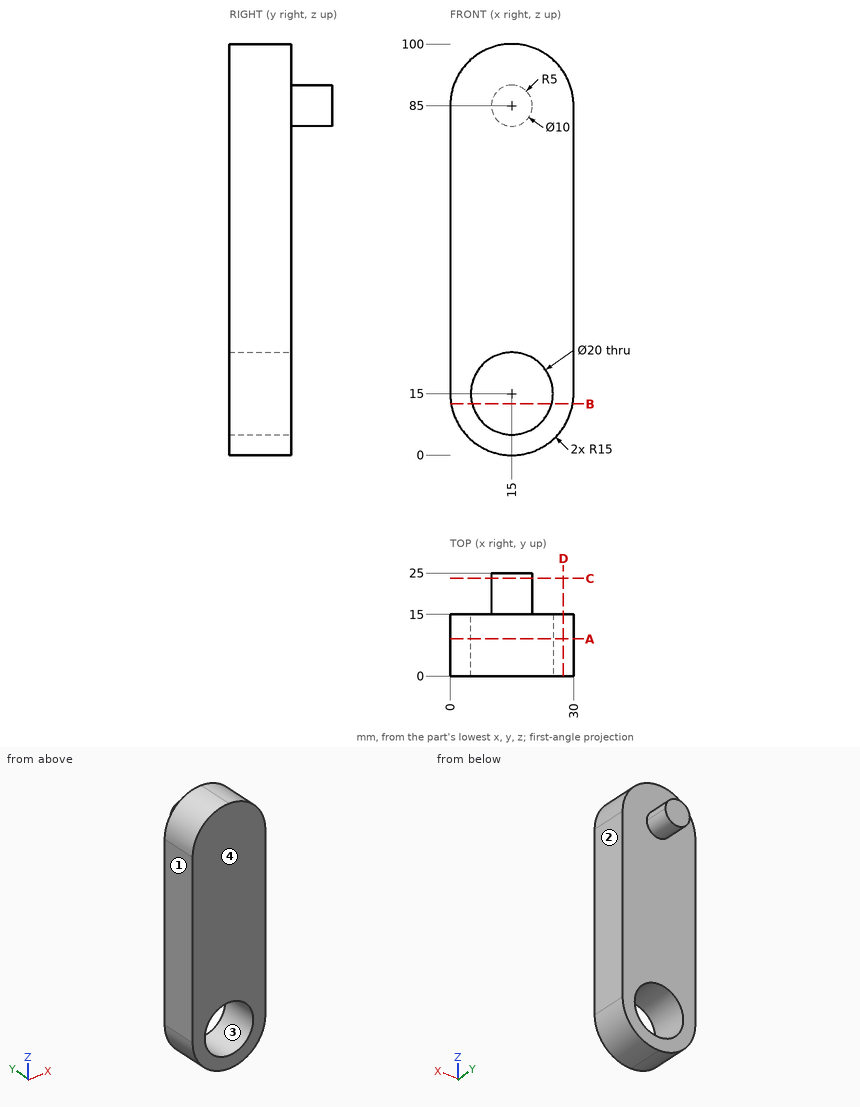
Job drawing, mm, ordinate dimensions from the low corner. One solid piece. Coordinates: 2 decimals unless noted, no trailing zeros. Write each loop counter-clockwise with the first axis right and the second up, starting at its lowest first coordinate (ties: lowest second). Pieces come first, ordered by that corner, then holes. Notation, with made-up numbers: (-36.75, 34.5) - (-24.75, 34.5) arc R34 cw to (-24.75, 69.5) - close; hole circle Ø1 at (18, -17.5). An arc over 180 degrees is marked (long way). Use a Markdown table: item, result. Add a question column.
Item 1: Band-saw the part on B-B, the plane z = 12.5. Give the cut face in (x, y), and give its area (3 significant figures).
Item 2: Flat gauge pins, fed straight in: pin 1 (5 mm diameter, centred on y = 19, z = 85.5, fed in from -X); pin 2 (1.5 mm diameter, centred on x = 18, y = 18, fed in from -Z); pin 3 (1.5 mm diameter, centred on x = 20, y = 13, fed in from +Z); pin 4 (18 mm diameter, centred on x = 15, z = 15, fed in from +Y). Where does each tip first touch, or does it go through?
Item 3: Mould opens along X. For the marked faces 1, 2, 3 and 4 say: pulls with the +X half, pulls with the -X half, needs draft (parallel to the pull), parting line crosses it, or undercut.
Item 4: Band-saw the part on A-A, the plane y = 9. Give the cut face in (x, z).
Item 5: Drill centre lines: L1, parallel to Y at x = 12, z = 32.5; L2, parallel to X at y = 8.75, z = 20.5; L3, parallel to Z at x = 20.5, y = 2. Where is each one in solid material? Low to high. Write a range as from..to.
Item 6: Band-saw the part on C-C, the plane y = 23.75. Give the cut face in (x, z).
Item 7: Band-saw the part on D-D, the plane x = 27.5. Give the cut face in (y, z), and give its area (3 significant figures).
Numbers:
| question | item | result |
|---|---|---|
| 1 | outline | (0.21, 0) - (5.32, 0) - (5.32, 15) - (0.21, 15) - close; (24.68, 0) - (29.79, 0) - (29.79, 15) - (24.68, 15) - close |
| 1 | area | 153 mm2 |
| 2 | pin 1 | x = 10 |
| 2 | pin 2 | z = 80.53 |
| 2 | pin 3 | z = 99.39 |
| 2 | pin 4 | through |
| 3 | face 1 | pulls with the -X half |
| 3 | face 2 | pulls with the +X half |
| 3 | face 3 | undercut |
| 3 | face 4 | needs draft |
| 4 | outline | (0, 15) arc R15 ccw to (15, 0) arc R15 ccw to (30, 15) - (30, 85) arc R15 ccw to (15, 100) arc R15 ccw to (0, 85) - close; hole circle Ø20 at (15, 15) |
| 5 | L1 | 0..15 |
| 5 | L2 | 0..6.65, 23.35..30 |
| 5 | L3 | 1.04..6.65, 23.35..98.96 |
| 6 | outline | circle Ø10 at (15, 85) |
| 7 | outline | (0, 6.71) - (15, 6.71) - (15, 93.29) - (0, 93.29) - close |
| 7 | area | 1,300 mm2 |
